Could you check a few things on this drawing? It's one solid part, dimensions in mm from its lowest x, y, z. Round coordinates to 2 decimals unless told otherwise and drop trailing zeros. Write each loop counter-clockwise with the first axis right and the second up, starting at its lowest first coordinate (ties: lowest second). Pieces come first, ordered by that corner, then holes. Notation, with made-up numbers: M 82.25,23 L 138.25,23 A16 cw 138.25,42 Z; hole C 22,3.5 d6. An arc over 180 degrees is marked long. One line per item, written item: value. Start each with the question number.
(1) I'm going to push flat-ended pins straight in: pin 1 Ø1 at (y, z) = (13, 4) entering from +X; pin 2 Ø3 at (y, z) = (13.5, 2.5) entering from +X; pin 3 Ø1 at (y, z) = (20, 2) entering from -X. Where does each tip first touch, or does it pass through?
(2) I want a section at B-B on x = 4.5. Please give me the cut outline in (y, z), and give its area (3 significant figures).
(3) If I drill on L1, parallel to Y at x = 36, z = 4.7; L2, parallel to Y at x = 19.5, z = 3.8; L3, parallel to X at y = 5, z = 2.6, over which ranges is the centre line in solid material (lowest first)?
(4) I want a section at A-A on z = 1.2. Please give me the cut outline in (x, y).
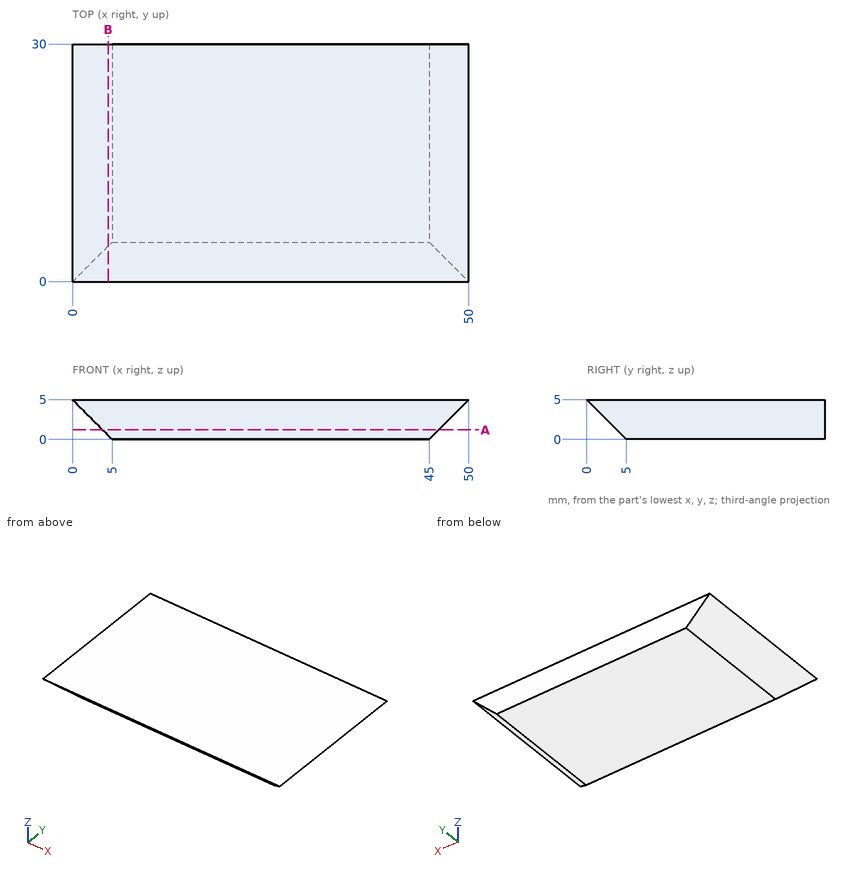
Found:
1. pin 1: stops at x = 49.5
1. pin 2: stops at x = 49
1. pin 3: stops at x = 2.5
2. outline: M 0,5 L 4.5,0.5 L 30,0.5 L 30,5 Z
2. area: 125 mm²
3. L1: y = 0.3 to 30
3. L2: y = 1.2 to 30
3. L3: x = 2.4 to 47.6
4. outline: M 3.8,3.8 L 46.2,3.8 L 46.2,30 L 3.8,30 Z
